Part model, mm, in its own coordinate system. Face numbers are marked on the shaded views. A direction names the side the tool comes from. Coordinates: 2 decimals unless noted, no trailing zeros. Order: outer loops, then holes, each group sorted by start corner. A loop starts at its lowest first (then second) coordinate and runs counter-clockwise, first axis right, second up. Notation, with made-up numbers: (64, 87) - (68, 87) arc R23 ccw to (68, 113) - close; hole circle Ø2 at (86.25, 26). An arc over 180 degrees is marked (long way). Use a Markdown table: item, result. Add a question column.
1) Tool access for the marked faces 4, 5 and 6: list every direction of +Z, -Z, +X, -X, +Y, -Y with a clear straight run to the whole face (end or side of a thin tool).
2) Saw through at C-C on y = -63.5. List the corners of the cut face in (x, z), then the cut area to 3 significant figures.
3) Drop flat-ended pins along their axis: P1, Ø3, axis at x = 36, z = 293, coming from the -Y side; P2, Ø3, axis at x = -52.5, y = -8.5, coming from the +Z side; P3, Ø1, axis at y = 42.5, z = 184, coming from the -X side. Give the stop position or say it passes through.
4) Saw through at B-B on z = -178.5. List the corners of the cut face in (x, y).
5) Two-plate mould, pull along Z, no slides. Class the marked faces 1, 2 and 3: +Z half, -Z half, draft (parallel to the pull), parting line (faces both ways), or undercut.
6) Wall check: L1, parallel to Y at x = 0, z = -228.75; L2, parallel to Y at x = 0, z = -248.75; L3, parallel to Z at x = -87, y = 48. Give the ranges that are in metal, low to high. Write a range as [from, to].
7) Saw through at D-D on z = 247. List the corners of the cut face in (x, y), then the cut area to 3 significant figures.
```python
from build123d import *

# Parameters (mm, degrees)
SKETCH3_R           = 10
BOSS_EXTRUDE3_DEPTH = 5
SKETCH16_R          = 7.5
BOSS_EXTRUDE7_DEPTH = 40
SKETCH19_R          = 4
CUT_EXTRUDE3_DEPTH  = 40
SKETCH20_R          = 10
BOSS_EXTRUDE8_DEPTH = 5
SKETCH21_W          = 10.753504306
SKETCH21_H          = 13.699669868
BOSS_EXTRUDE9_DEPTH = 20
CUT_EXTRUDE5_DEPTH  = 16.376752153
SKETCH25_R          = 3
CUT_EXTRUDE6_DEPTH  = 16.376752153
CUT_EXTRUDE7_DEPTH  = 10
SKETCH28_W          = 0.376752153
SKETCH28_H          = 3.904338954
CUT_EXTRUDE8_DEPTH  = 8.338161
SCALE1_SCALE        = 10


with BuildPart() as part:
    # Sketch3 → Boss-Extrude3 (new body)
    with BuildSketch(Plane.XY):
        Circle(SKETCH3_R)
    extrude(amount=BOSS_EXTRUDE3_DEPTH)

    # Sketch14 → CBORE for M4 Cheese Head Screw1 (revolve, cut)
    with BuildSketch(Plane(origin=(0, 0, 5), x_dir=(0, -1, 0), z_dir=(1, 0, 0))):
        Polygon((0, 0), (0, 8.942065486), (2.4, 7.5), (2.4, 2.6), (4, 2.6), (4, 0.025), (4.025, 0), align=None)
    revolve(axis=Axis((0, 0, 11.35), (0, 0, -1)), mode=Mode.SUBTRACT)

    # Sketch16 → Boss-Extrude7 (add)
    with BuildSketch(Plane.XY.offset(5)):
        Circle(SKETCH16_R)
    extrude(amount=BOSS_EXTRUDE7_DEPTH)

    # Sketch19 → Cut-Extrude3 (cut)
    with BuildSketch(Plane.XY.offset(45)):
        Circle(SKETCH19_R)
    extrude(amount=-CUT_EXTRUDE3_DEPTH, mode=Mode.SUBTRACT)

    # Sketch20 → Boss-Extrude8 (add)
    with BuildSketch(Plane.XY.offset(45)):
        Circle(SKETCH20_R)
    extrude(amount=BOSS_EXTRUDE8_DEPTH)

    # Sketch21 → Boss-Extrude9 (add)
    with BuildSketch(Plane.XY.offset(50)):
        Rectangle(SKETCH21_W, SKETCH21_H)
    extrude(amount=BOSS_EXTRUDE9_DEPTH)

    # Sketch24 → Cut-Extrude5 (cut, through all)
    with BuildSketch(Plane(origin=(5.376752153, 0, 0), x_dir=(0, 0, -1), z_dir=(1, 0, 0))):
        with BuildLine():
            Line((-58.338160712, 1.952169477), (-50, 1.952169477))
            Line((-50, 1.952169477), (-50, 6.849834934))
            Line((-50, 6.849834934), (-70, 6.849834934))
            Line((-70, 6.849834934), (-70, 0))
            ThreePointArc((-70, 0), (-67.509703972, 4.324509912), (-62.51944561, 4.34129588))
            Line((-62.51944561, 4.34129588), (-58.338160712, 1.952169477))
        make_face()
        with BuildLine():
            Line((-50, -6.849834934), (-50, -1.952169477))
            Line((-50, -1.952169477), (-58.338160712, -1.952169477))
            Line((-58.338160712, -1.952169477), (-62.51944561, -4.34129588))
            ThreePointArc((-62.51944561, -4.34129588), (-67.509703972, -4.324509912), (-70, 0))
            Line((-70, 0), (-70, -6.849834934))
            Line((-70, -6.849834934), (-50, -6.849834934))
        make_face()
    extrude(amount=-CUT_EXTRUDE5_DEPTH, mode=Mode.SUBTRACT)

    # Sketch25 → Cut-Extrude6 (cut, through all)
    with BuildSketch(Plane(origin=(5.376752153, 0, 0), x_dir=(0, 0, -1), z_dir=(1, 0, 0))):
        with Locations((-65, 0)):
            Circle(SKETCH25_R)
    extrude(amount=-CUT_EXTRUDE6_DEPTH, mode=Mode.SUBTRACT)

    # Sketch27 → Cut-Extrude7 (cut, symmetric)
    with BuildSketch(Plane(origin=(0, 1.952169477, 0), x_dir=(1, 0, 0), z_dir=(0, 1, 0))):
        Polygon((5, -58.338160712), (5, -71.045531856), (7.637324511, -71.045531856), (7.637324511, -50), (5.376752153, -50), (5.376752153, -58.338160712), align=None)
        Polygon((-8.147357924, -71.045531856), (-5, -71.045531856), (-5, -58.338160712), (-5.376752153, -58.338160712), (-5.376752153, -50), (-8.147357924, -50), align=None)
    extrude(amount=CUT_EXTRUDE7_DEPTH, both=True, mode=Mode.SUBTRACT)

    # Sketch28 → Cut-Extrude8 (cut)
    with BuildSketch(Plane.XY.offset(58.338160712)):
        with Locations((-5.188376076, 0)):
            Rectangle(SKETCH28_W, SKETCH28_H)
        with Locations((5.188376076, 0)):
            Rectangle(SKETCH28_W, SKETCH28_H)
    extrude(amount=-CUT_EXTRUDE8_DEPTH, mode=Mode.SUBTRACT)


with BuildPart() as part_1:
    # Scale1: scaled about (0, 0, 29.145316633)
    add(part.part.scale(SCALE1_SCALE).moved(Location((0, 0, -262.307849697))))


solid = part_1.part
```
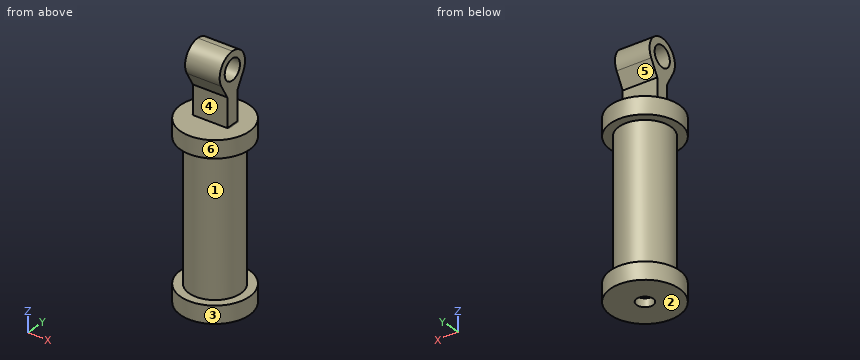
Results are:
| question | item | result |
|---|---|---|
| 1 | face 4 | +X, -X, -Y |
| 1 | face 5 | +X, -X, +Y |
| 1 | face 6 | +Z, -Z |
| 2 | outline | (-77.25, -262.31) - (77.25, -262.31) - (77.25, -212.31) - (39.91, -212.31) - (39.91, 187.69) - (77.25, 187.69) - (77.25, 237.69) - (-77.25, 237.69) - (-77.25, 187.69) - (-39.91, 187.69) - (-39.91, -212.31) - (-77.25, -212.31) - close |
| 2 | area | 47,400 mm2 |
| 3 | P1 | y = -19.52 |
| 3 | P2 | z = 237.69 |
| 3 | P3 | x = -62.14 |
| 4 | outline | circle Ø150 at (0, 0); hole circle Ø80 at (0, 0) |
| 5 | face 1 | undercut |
| 5 | face 2 | -Z half |
| 5 | face 3 | draft |
| 6 | L1 | [-100, -40], [40, 100] |
| 6 | L2 | [-100, -24], [24, 100] |
| 6 | L3 | [-262.31, -212.31], [187.69, 237.69] |
| 7 | outline | (-50, -19.52) - (50, -19.52) - (50, 19.52) - (-50, 19.52) - close |
| 7 | area | 3,900 mm2 |
